Could you check a few things on this model? Use its own coordinates, in mm. A direction names the side the tool comes from. Coordinates: 2 decimals unless noted, no trailing zeros. Loops run counter-clockwise (first coordinate to the right, second up) from the corner with the lowest first, then second, coordinate; pieces in that order, holes last. Notation, with made-up numbers: (-25.5, -37) -> (11.5, -37) arc R34 ccw to (11.5, -2) -> close; hole circle Ø3 at (15, 21.5). An arc over 180 degrees is marked (long way). One line per question, with ' | ' between items.
from build123d import *

# Parameters (mm, degrees)
SKETCH_R     = 1.5
SKETCH_R_2   = 1.1
PAD_DEPTH    = 3
FILLET_R     = 2.6
SKETCH001_W  = 6
SKETCH001_H  = 40
SKETCH001_R  = 1.5
PAD001_DEPTH = 3
FILLET001_R  = 2.5
CHAMFER_SIZE = 5
FILLET002_R  = 2


with BuildPart() as part:
    # Sketch → Pad (new body)
    with BuildSketch(Plane.XY):
        Polygon((-22.7, 0), (-22.7, 5.4), (-35, 5.4), (-35, -7), (35, -7), (35, 5.4), (22.7, 5.4), (22.7, 0), align=None)
        with Locations((-7.5, -3.5)):
            Circle(SKETCH_R, mode=Mode.SUBTRACT)
        with Locations((7.5, -3.5)):
            Circle(SKETCH_R, mode=Mode.SUBTRACT)
        with Locations((-25.4, 2.7)):
            Circle(SKETCH_R_2, mode=Mode.SUBTRACT)
        with Locations((25.4, 2.7)):
            Circle(SKETCH_R_2, mode=Mode.SUBTRACT)
    extrude(amount=PAD_DEPTH)

    # Fillet
    fillet_edges = [part.edges().sort_by_distance(p)[0] for p in [
        (-22.7, 5.4, 1.5),
        (22.7, 5.4, 1.5),
    ]]
    fillet(fillet_edges, radius=FILLET_R)

    # Sketch001 → Pad001 (new body)
    with BuildSketch(Plane.XY.offset(3)):
        with Locations((-32, 0)):
            Rectangle(SKETCH001_W, SKETCH001_H)
        with Locations((-32, 17)):
            Circle(SKETCH001_R, mode=Mode.SUBTRACT)
        with Locations((-32, -17)):
            Circle(SKETCH001_R, mode=Mode.SUBTRACT)
        with Locations((32, 0)):
            Rectangle(SKETCH001_W, SKETCH001_H)
        with Locations((32, 17)):
            Circle(SKETCH001_R, mode=Mode.SUBTRACT)
        with Locations((32, -17)):
            Circle(SKETCH001_R, mode=Mode.SUBTRACT)
    extrude(amount=-PAD001_DEPTH)

    # Fillet001
    fillet001_edges = [part.edges().sort_by_distance(p)[0] for p in [
        (-35, -20, 1.5),
        (-29, -20, 1.5),
        (29, -20, 1.5),
        (35, -20, 1.5),
        (35, 20, 1.5),
        (29, 20, 1.5),
        (-29, 20, 1.5),
        (-35, 20, 1.5),
    ]]
    fillet(fillet001_edges, radius=FILLET001_R)

    # Chamfer
    chamfer_edges = [part.edges().sort_by_distance(p)[0] for p in [
        (-29, -7, 1.5),
        (29, -7, 1.5),
    ]]
    chamfer(chamfer_edges, length=CHAMFER_SIZE)

    # Fillet002
    fillet002_edges = [part.edges().sort_by_distance(p)[0] for p in [
        (-29, 5.4, 1.5),
        (-22.7, 0, 1.5),
        (22.7, 0, 1.5),
        (29, 5.4, 1.5),
    ]]
    fillet(fillet002_edges, radius=FILLET002_R)


solid = part.part
1) I need wall thicknesses on line 1 along Y through (x, z) = (32, 2.05); line 2 along Y through (x, z) = (-7.5, 0.85); line 3 along X through (y, z) = (-17.5, 0.45). Which ranges of each line are inside material? Lowest first, please. Write a range as from..to.
Data:
line 1: -20..-18.5, -15.5..15.5, 18.5..20 | line 2: -7..-5, -2..0 | line 3: -35..-33.41, -30.59..-29, 29..30.59, 33.41..35
2) On a 3-axis mill with a long thin cutter (end or side, diameter ignored), from which of +Z, -Z, +X, -X, +Y, -Y can I reach the whole of each face in a straight line? I mean faces 4 (the face through (26, 5.4, 1)), 5 (the face through (27, -10, 2)), 6 (the face through (35, 0, 1)). Say none if no direction works.
Data:
face 4: +Z, -Z, +Y | face 5: +Z, -Z, -Y | face 6: +Z, -Z, +X, +Y, -Y
3) If we section it at A-A on x = -7.5: Please give me the cut outline in (y, z).
Data:
outline: (-7, 0) -> (-5, 0) -> (-5, 3) -> (-7, 3) -> close; (-2, 0) -> (0, 0) -> (0, 3) -> (-2, 3) -> close
4) If we section it at B-B on z = 2.05: Give the number of separate pieces and of enclosed holes in the cut face, and give its area (3 significant figures).
Data:
separate pieces: 1 | enclosed holes: 8 | area: 919 mm²
5) If we section it at C-C on x = 11: Please give me the cut outline in (y, z), and give its area (3 significant figures).
Data:
outline: (-7, 0) -> (0, 0) -> (0, 3) -> (-7, 3) -> close | area: 21.0 mm²
6) We'd pull the mould along Y, two halves only. Please class faces 1 (the face through (34.287, -19.248, 1.479)), 2 (the face through (6.39, -2.49, 1.48)), 3 (the face through (34.248, 19.287, 1.479)): pulls with the +Y half, pulls with the -Y half, needs draft (parallel to the pull), parting line crosses it, or undercut.
Data:
face 1: pulls with the -Y half | face 2: undercut | face 3: pulls with the +Y half
7) I'm going to push flat-ended pins straight in: pin 1 Ø12 at (x, y) = (12.5, 9) entering from +Z; pin 2 Ø0.9 at (x, z) = (2.5, 2) entering from +Y; pin 3 Ø0.9 at (x, z) = (-26, 1.5) entering from +Y. Where does each tip first touch, or does it pass through?
Data:
pin 1: through | pin 2: y = 0 | pin 3: y = 5.4
